```python
from build123d import *

# Parameters (mm, degrees)
BOSS_EXTRUDE4_DEPTH  = 6.746875
SKETCH6_R            = 3.96875
BOSS_EXTRUDE5_DEPTH  = 6.746875
SHELL2_T             = -0.79375
BOSS_EXTRUDE6_REACH  = 19.089
CUT_EXTRUDE2_START   = -0.396875
SKETCH11_R           = 3.96875
CUT_EXTRUDE2_DEPTH   = 0.396875
SKETCH13_R           = 3.96875
BOSS_EXTRUDE11_DEPTH = 6.35
SKETCH14_R           = 2.38125
CUT_EXTRUDE3_DEPTH   = 1.984375
CUT_EXTRUDE4_DEPTH   = 3.571875
SKETCH17_R           = 1.190625
CUT_EXTRUDE5_DEPTH   = 2.38125
SKETCH18_W           = 8.89
SKETCH18_H           = 15.24
CUT_EXTRUDE6_DEPTH   = 12.7


with BuildPart() as part:
    # Sketch2 → Boss-Extrude4 (new body)
    with BuildSketch(Plane(origin=(0, 0, 0), x_dir=(0, 0, -1), z_dir=(1, 0, 0))):
        Polygon((-4.365625, 0), (4.365625, 0), (4.365625, 11.1125), (-1.984375, 11.1125), (-1.984375, 3.175), (-4.365625, 3.175), align=None)
    extrude(amount=BOSS_EXTRUDE4_DEPTH)

    # Sketch6 → Boss-Extrude5 (add)
    with BuildSketch(Plane(origin=(6.746875, 0, 0), x_dir=(0, 0, -1), z_dir=(1, 0, 0))):
        with Locations((0.396875, 11.1125)):
            Circle(SKETCH6_R)
    extrude(amount=-BOSS_EXTRUDE5_DEPTH)

    # Shell2
    shell2_openings = [part.faces().sort_by_distance(p)[0] for p in [
        (3.3734375, 0, 0),
    ]]
    offset(amount=SHELL2_T, openings=shell2_openings, kind=Kind.INTERSECTION)

    # Sketch7 → Boss-Extrude6 (add, up to next)
    with BuildSketch(Plane.XZ, mode=Mode.PRIVATE) as boss_extrude6_sk1:
        Polygon((5.953125, 3.571875), (5.953125, 2.38125), (1.190625, 2.38125), (1.190625, -2.38125), (5.953125, -2.38125), (5.953125, -3.571875), (0.79375, -3.571875), (0.79375, 3.571875), align=None)
    boss_extrude6_tool1 = extrude(boss_extrude6_sk1.sketch, amount=-BOSS_EXTRUDE6_REACH, mode=Mode.PRIVATE) - part.part
    add(boss_extrude6_tool1.solids().sort_by_distance((5.865004, 0, 2.976562))[0])

    # Sketch11 → Cut-Extrude2 (cut)
    with BuildSketch(Plane.ZY.offset(CUT_EXTRUDE2_START)):
        with Locations((-0.396875, 11.1125)):
            Circle(SKETCH11_R)
    extrude(amount=CUT_EXTRUDE2_DEPTH, mode=Mode.SUBTRACT)

    # Sketch13 → Boss-Extrude11 (add)
    with BuildSketch(Plane(origin=(6.746875, 0, 0), x_dir=(0, 0, -1), z_dir=(1, 0, 0))):
        with Locations((0.396875, 11.1125)):
            Circle(SKETCH13_R)
    extrude(amount=-BOSS_EXTRUDE11_DEPTH)

    # Sketch14 → Cut-Extrude3 (cut)
    with BuildSketch(Plane(origin=(0, 0, -4.365625), x_dir=(-1, 0, 0), z_dir=(0, 0, -1))):
        with Locations(Location((-3.571875, 3.96875, 0), (0, 0, 90))):
            Circle(SKETCH14_R)
        with Locations(Location((-3.571875, 11.90625, 0), (0, 0, 340.528779366))):
            Circle(SKETCH14_R)
    extrude(amount=-CUT_EXTRUDE3_DEPTH, mode=Mode.SUBTRACT)

    # Sketch16 → Cut-Extrude4 (cut)
    with BuildSketch(Plane(origin=(0, 0, -2.38125), x_dir=(-1, 0, 0), z_dir=(0, 0, -1))):
        with BuildLine():
            Line((-2.778125, 9.66118597), (-2.778125, 14.15131403))
            ThreePointArc((-2.778125, 14.15131403), (-5.953125, 11.90625), (-2.778125, 9.66118597))
        make_face()
    extrude(amount=-CUT_EXTRUDE4_DEPTH, mode=Mode.SUBTRACT)

    # Sketch17 → Cut-Extrude5 (cut)
    with BuildSketch(Plane.ZY.offset(-0.396875)):
        with Locations((-0.396875, 11.1125)):
            Circle(SKETCH17_R)
    extrude(amount=-CUT_EXTRUDE5_DEPTH, mode=Mode.SUBTRACT)

    # Mirror6: part across plane


with BuildPart() as part_1:
    add(part.part)
    add(part.part.mirror(Plane(origin=(0, 0, 0), x_dir=(0, 0, 1), z_dir=(1, 0, 0))))

    # Sketch18 → Cut-Extrude6 (cut)
    with BuildSketch(Plane(origin=(0, 0, 0), x_dir=(0, 0, -1), z_dir=(1, 0, 0))):
        with Locations((0.079375, 7.62)):
            Rectangle(SKETCH18_W, SKETCH18_H)
    extrude(amount=CUT_EXTRUDE6_DEPTH, mode=Mode.SUBTRACT)


solid = part_1.part
```
The listing builds one solid part. Answer for the finished solid, in the listing's coordinates (mm). A direction names the side the tool comes from. Coordinates: 2 decimals unless noted, no trailing zeros. Loops run counter-clockwise (first coordinate to the right, second up) from the corner with the lowest first, then second, coordinate; pieces in that order, holes last. Notation, with made-up numbers: (2, -11.5) -> (44, -11.5) arc R20 cw to (44, 16.5) -> close; hole circle Ø8 at (-10.75, 36). An arc over 180 degrees is marked (long way). Return JSON: item names as keys, results as strings. Group by question number.
(1) Which of the six approach directions +Z, -Z, +X, -X, +Y, -Y give full straight-line access (tool end or side, diameter ignored) to faces 4 (the flat face through (-1, 0, 0)), 5 (the cylindrical face through (-1.57, 9.95, -0.65)), 6 (the flat face through (0, 3, -1)), 7 (the flat face through (-2.778, 12.4, -1)), 8 (the flat face through (-4, 1, -2.381))?
(2) A cutting plane is placed at A-A on x = -5.5. Write down the section's boundary in (y, z) (1 decimal).
(3) Determine the mould class of faces 1 (the flat face through (-0.397, 11, 1)), 2 (the cylindrical face through (-0.201, 7.591, -2.227)), 3 (the cylindrical face through (-4.29, 6.24, -3.39)) for opening direction X: released by +X, released by -X, zero draft, split by the parting line, or undercut.
(4) A cutting plane is placed at C-C on z = -2.75. Write down the section's boundary in (x, y).
(5) A cutting plane is placed at D-D on y = 9. Write down the section's boundary in (x, z).
(6) A cutting plane is placed at B-B on z = -1.75. Write down the section's boundary in (x, y).
(7) Given pin 1 Ø1.2 at (x, z) = (-4.5, 3) entering from +Y; pin 2 Ø4 at (x, y) = (-3.5, 7.5) entering from +Z; pin 3 Ø0.5 at (x, y) = (-2.5, 11.5) entering from -Z, each flat-ended and moving along its own axis, determine where each tip first touches the part or whether it passes through.
(8) Find the intervals of material crossed by probe 1 along X at (y, z) = (1.5, 0.75); probe 2 along Y at (x, z) = (-2.5, -0.5); probe 3 along Z at (x, y) = (-2.25, 6.5), in increasing order. Write a range as from..to.
The answers:
{
 "1": {"face 4": "+Z, -Z, +X, -X, -Y", "face 5": "+X", "face 6": "+Z, -Z, +X, +Y, -Y", "face 7": "-Z", "face 8": "-Y"},
 "2": {"outline": "(0, -4.4) -> (2.6, -4.4) -> (2.6, -2.4) -> (0, -2.4) -> close; (0, 2.4) -> (2.4, 2.4) -> (2.4, 1.2) -> (7.5, 1.2) arc R4 ccw to (7.7, -2.4) -> (5.4, -2.4) -> (5.4, -4.4) -> (10.5, -4.4) -> (10.5, 1.2) -> (13.3, 1.2) -> (13.3, -3.7) arc R4 ccw (long way) to (7.9, 2) -> (3.2, 2) -> (3.2, 4.4) -> (0, 4.4) -> close"},
 "3": {"face 1": "released by +X", "face 2": "zero draft", "face 3": "undercut"},
 "4": {"outline": "(-6.75, 0) -> (0, 0) -> (0, 7.92) -> (-0.4, 7.92) -> (-0.4, 14.31) -> (-6.75, 14.31) -> close; hole circle Ø4.76 at (-3.57, 3.97); hole circle Ø4.76 at (-3.57, 11.91)"},
 "5": {"outline": "(-6.75, -4.37) -> (0, -4.37) -> (0, -3.76) -> (-0.4, -3.76) -> (-0.4, 2.96) -> (-6.75, 2.96) -> close"},
 "6": {"outline": "(-6.75, 0) -> (-5.95, 0) -> (-5.95, 7.38) -> (-1.19, 7.38) -> (-1.19, 0) -> (0, 0) -> (0, 7.38) -> (-0.4, 7.38) -> (-0.4, 14.84) -> (-6.75, 14.84) -> close; hole (-2.78, 9.66) -> (-2.78, 14.15) arc R2.38 ccw (long way) to start"},
 "7": {"pin 1": "stops at y = 13.93", "pin 2": "stops at z = 3.23", "pin 3": "stops at z = -2.38"},
 "8": {"probe 1": "x = -6.75..-5.95, -1.19..0", "probe 2": "y = 7.15..9.93, 12.3..15.08", "probe 3": "z = -4.37..-2.38, 1.19..1.98"}
}
